Drawing for the job (mm, zero at the part's lowest x, y, z). Round coordinates to 2 decimals unless told otherwise and drop trailing zeros. Loops run counter-clockwise (first coordinate to the right, second up) from the corner with the lowest first, then second, coordinate; pieces in that order, holes last. Notation, with made-up numbers: M 83,84 L 137,84 A11 ccw 137,103 Z; hole C 48.25,-28.5 d9. An arc over 180 degrees is marked long. Put each result on its own line as item: value. Start each with the question number.
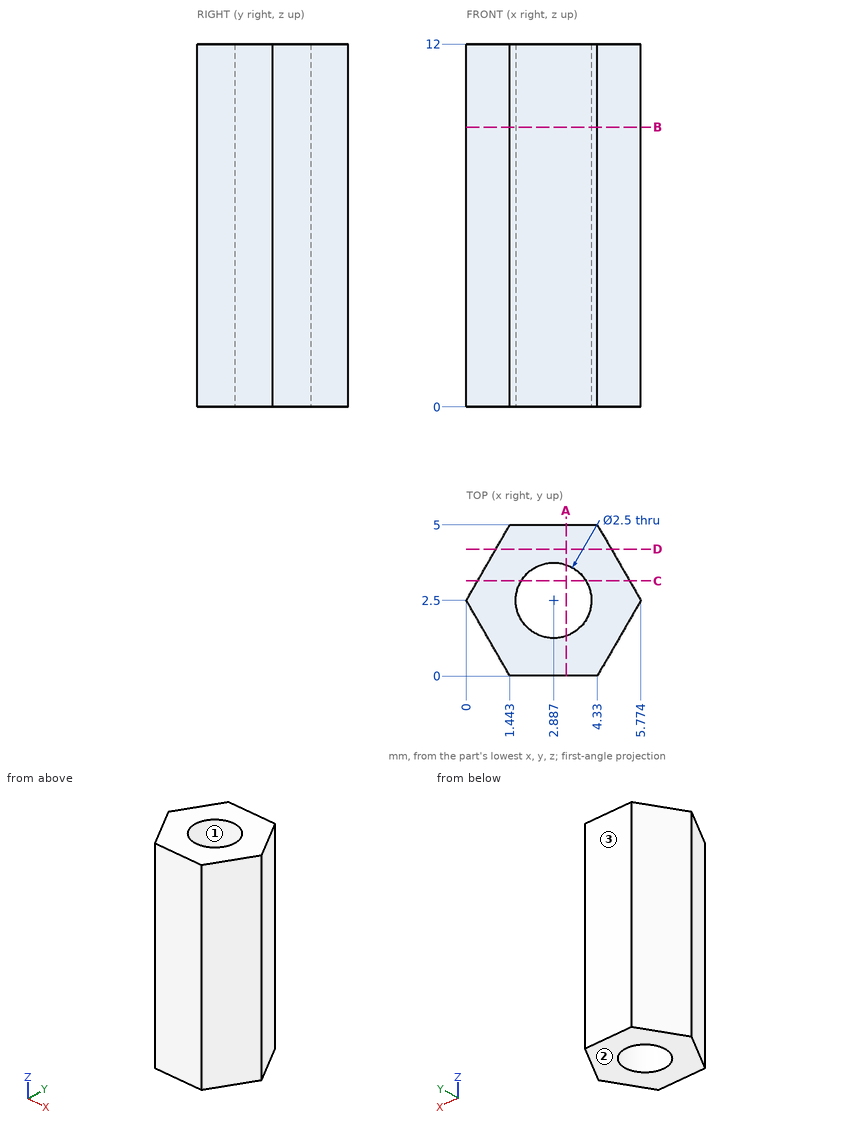
1. Mould opens along Y. For the marked faces 1, 2 and 3 say: released by +Y, released by -Y, zero draft, split by the parting line, or undercut.
2. Cut at A-A, the plane x = 3.3. Give the cut face in (y, z).
3. Cut at C-C, the plane y = 3.15. Give the cut face in (x, z) (1 decimal).
4. Cut at D-D, the plane y = 4.2. Give the cut face in (x, z).
5. Wall check: L1, parallel to Y at x = 2.7, z = 4.75 (1 decimal); L2, parallel to X at y = 2.7, z = 7 (1 decimal); L3, parallel to X at y = 3.3, z = 4.5 (1 decimal). Give the ranges that are in metal, low to high.
6. Cut at B-B, the plane z = 9.25. Give the cut face in (x, y).
Results list:
1. face 1: undercut
1. face 2: zero draft
1. face 3: released by +Y
2. outline: M 0,0 L 1.32,0 L 1.32,12 L 0,12 Z; M 3.68,0 L 5,0 L 5,12 L 3.68,12 Z
3. outline: M 0.4,0 L 1.8,0 L 1.8,12 L 0.4,12 Z; M 4,0 L 5.4,0 L 5.4,12 L 4,12 Z
4. outline: M 0.98,0 L 4.79,0 L 4.79,12 L 0.98,12 Z
5. L1: y = 0 to 1.3, 3.7 to 5
5. L2: x = 0.1 to 1.7, 4.1 to 5.7
5. L3: x = 0.5 to 1.9, 3.8 to 5.3
6. outline: M 0,2.5 L 1.44,0 L 4.33,0 L 5.77,2.5 L 4.33,5 L 1.44,5 Z; hole C 2.89,2.5 d2.5
